Here's how the part is built. I have some questions about the finished solid (model axes, mm). A direction names the side the tool comes from. Round coordinates to 2 decimals unless told otherwise and drop trailing zeros. Order: outer loops, then holes, each group sorted by start corner. A loop starts at its lowest first (then second) coordinate and runs counter-clockwise, first axis right, second up. Notation, with made-up numbers: M -1,-27 L 43,-27 A16 cw 43,4 Z; hole C 84.25,30 d2. An arc over 180 degrees is marked long. Write item = value, one per line. Start each with the question number.
Item 1: I want a section at B-B, the plane y = 3.25. List the corners of the cut face in (x, z) for me.
Item 2: Please list where these lines run through material, in increasing order: L1, parallel to X at y = 0.25, z = -0.25; L2, parallel to X at y = 2.25, z = -4.4; L3, parallel to Z at x = 7.5, y = 3.75.
Item 3: I want a section at A-A, the plane y = -0.5. List the corners of the cut face in (x, z) for me.
Item 4: I want a section at C-C, the plane x = 6.5. List the corners of the cut face in (y, z) for me, plus the area to 3 significant figures.
Item 5: I'm going to push flat-ended pins straight in: P1, Ø0.7, axis at x = 5, y = -0.5, coming from the -Z side; P2, Ø0.7, axis at y = -2, z = -2.5, coming from the +X side. Where does each tip first touch, or does it pass through?
Item 6: We'd pull the mould along Z, two halves only. Please class faces 3 (the face through (9.1, 5, -3)), 4 (the face through (5, 3, 0)), 5 (the face through (1, 0, -3)): pulls with the +Z half, pulls with the -Z half, needs draft (parallel to the pull), parting line crosses it, or undercut.
Item 7: I want a section at D-D, the plane z = -3.8. List the corners of the cut face in (x, y) for me.
Item 8: For faces 1 (the face through (5, 4, -0.8)), 2 (the face through (5, 3, -5.75)), which set-ups out of +Z, -Z, +X, -X, +Y, -Y let a thin tool reach every point of the face, with its end or its side?
```python
from build123d import *

# Parameters (mm, degrees)
SKETCH_1_W                         = 9.9
SKETCH_1_H                         = 5.75
EXTRUDE_1_DEPTH                    = 7
SKETCH_2_W                         = 8.3
SKETCH_2_H                         = 4.15
CUT_EXTRUDE_1_DEPTH                = 5
CUT_EXTRUDE_2_REACH                = 15.419
SKETCH_3_W                         = 1
SKETCH_3_H                         = 0.8
EXTRUDE_START                      = -5.5
SKETCH_4_W                         = 0.64
SKETCH_4_H                         = 0.64
EXTRUDE_2_DEPTH                    = 10.5
CHAMFER_1_SIZE                     = 0.2
PATTERN_LINEAR_4_COUNT             = 3
PATTERN_LINEAR_4_PITCH             = 2.5
CHAMFER_1_OF_PATTERN_LINEAR_4_SIZE = 0.2
CUT_EXTRUDE_3_REACH                = 15.419
CUT_EXTRUDE_4_DEPTH                = 14.419109508
FILLET_1_R                         = 0.1


with BuildPart() as part:
    # Эскиз1 → Бобышка-Вытянуть1 (new body)
    with BuildSketch(Plane(origin=(0, 0, 0), x_dir=(1, 0, 0), z_dir=(0, 1, 0))):
        with Locations((4.95, 2.875)):
            Rectangle(SKETCH_1_W, SKETCH_1_H)
    extrude(amount=EXTRUDE_1_DEPTH)

    # Эскиз2 → Вырез-Вытянуть1 (cut)
    with BuildSketch(Plane(origin=(0, 7, 0), x_dir=(1, 0, 0), z_dir=(0, 1, 0))):
        with Locations((4.95, 2.875)):
            Rectangle(SKETCH_2_W, SKETCH_2_H)
    extrude(amount=-CUT_EXTRUDE_1_DEPTH, mode=Mode.SUBTRACT)

    # Эскиз3 → Вырез-Вытянуть2 (cut, up to next)
    with BuildSketch(Plane.XY, mode=Mode.PRIVATE) as cut_extrude_2_sk1:
        with Locations((2.45, 0.4)):
            Rectangle(SKETCH_3_W, SKETCH_3_H)
    cut_extrude_2_tool1 = extrude(cut_extrude_2_sk1.sketch, amount=-CUT_EXTRUDE_2_REACH, mode=Mode.PRIVATE) & part.part
    # Эскиз3 → Вырез-Вытянуть2 (cut, up to next)
    with BuildSketch(Plane.XY, mode=Mode.PRIVATE) as cut_extrude_2_sk2:
        with Locations((4.95, 0.4)):
            Rectangle(SKETCH_3_W, SKETCH_3_H)
    cut_extrude_2_tool2 = extrude(cut_extrude_2_sk2.sketch, amount=-CUT_EXTRUDE_2_REACH, mode=Mode.PRIVATE) & part.part
    # Эскиз3 → Вырез-Вытянуть2 (cut, up to next)
    with BuildSketch(Plane.XY, mode=Mode.PRIVATE) as cut_extrude_2_sk3:
        with Locations((7.45, 0.4)):
            Rectangle(SKETCH_3_W, SKETCH_3_H)
    cut_extrude_2_tool3 = extrude(cut_extrude_2_sk3.sketch, amount=-CUT_EXTRUDE_2_REACH, mode=Mode.PRIVATE) & part.part
    add(cut_extrude_2_tool1.solids().sort_by_distance((2.45, 0.4, 0))[0], mode=Mode.SUBTRACT)
    add(cut_extrude_2_tool2.solids().sort_by_distance((4.95, 0.4, 0))[0], mode=Mode.SUBTRACT)
    add(cut_extrude_2_tool3.solids().sort_by_distance((7.45, 0.4, 0))[0], mode=Mode.SUBTRACT)

    # Эскиз4 → Бобышка-Вытянуть2 (add)
    with BuildSketch(Plane(origin=(0, 2, 0), x_dir=(1, 0, 0), z_dir=(0, 1, 0)).offset(EXTRUDE_START)):
        with Locations((2.45, 2.64)):
            Rectangle(SKETCH_4_W, SKETCH_4_H)
    extrude_2 = extrude(amount=EXTRUDE_2_DEPTH)

    # Фаска1
    chamfer_1_edges = [part.edges().sort_by_distance(p)[0] for p in [
        (2.13, 7, -2.64),
        (2.13, -3.5, -2.64),
        (2.45, 7, -2.96),
        (2.45, -3.5, -2.96),
        (2.77, 7, -2.64),
        (2.77, -3.5, -2.64),
        (2.45, 7, -2.32),
        (2.45, -3.5, -2.32),
    ]]
    chamfer(chamfer_1_edges, length=CHAMFER_1_SIZE)

    # Линейный массив4: Бобышка-Вытянуть2 ×3
    with Locations(*[(i * PATTERN_LINEAR_4_PITCH, 0, 0) for i in range(1, PATTERN_LINEAR_4_COUNT)]):
        add(extrude_2)

    # Фаска1 of Линейный массив4
    chamfer_1_of_pattern_linear_4_edges = [part.edges().sort_by_distance(p)[0] for p in [
        (4.63, 7, -2.64),
        (4.63, -3.5, -2.64),
        (4.95, 7, -2.96),
        (4.95, -3.5, -2.96),
        (5.27, 7, -2.64),
        (5.27, -3.5, -2.64),
        (4.95, 7, -2.32),
        (4.95, -3.5, -2.32),
        (7.13, 7, -2.64),
        (7.13, -3.5, -2.64),
        (7.45, 7, -2.96),
        (7.45, -3.5, -2.96),
        (7.77, 7, -2.64),
        (7.77, -3.5, -2.64),
        (7.45, 7, -2.32),
        (7.45, -3.5, -2.32),
    ]]
    chamfer(chamfer_1_of_pattern_linear_4_edges, length=CHAMFER_1_OF_PATTERN_LINEAR_4_SIZE)

    # Эскиз5 → Вырез-Вытянуть3 (cut, up to next)
    with BuildSketch(Plane.XY, mode=Mode.PRIVATE) as cut_extrude_3_sk1:
        with BuildLine():
            Line((1.95, 7), (2.95, 7))
            Line((2.95, 7), (2.95, 4))
            Line((2.95, 4), (2.45, 4))
            ThreePointArc((2.45, 4), (2.096446609, 4.146446609), (1.95, 4.5))
            Line((1.95, 4.5), (1.95, 6.153589838))
            ThreePointArc((1.95, 6.153589838), (1.976794919, 6.253589838), (2.05, 6.326794919))
            ThreePointArc((2.05, 6.326794919), (2.15, 6.5), (2.05, 6.673205081))
            ThreePointArc((2.05, 6.673205081), (1.976794919, 6.746410162), (1.95, 6.846410162))
            Line((1.95, 6.846410162), (1.95, 7))
        make_face()
    cut_extrude_3_tool1 = extrude(cut_extrude_3_sk1.sketch, amount=-CUT_EXTRUDE_3_REACH, mode=Mode.PRIVATE) & part.part
    # Эскиз5 → Вырез-Вытянуть3 (cut, up to next)
    with BuildSketch(Plane.XY, mode=Mode.PRIVATE) as cut_extrude_3_sk2:
        with BuildLine():
            Line((6.95, 7), (7.95, 7))
            Line((7.95, 7), (7.95, 6.846410162))
            ThreePointArc((7.95, 6.846410162), (7.923205081, 6.746410162), (7.85, 6.673205081))
            ThreePointArc((7.85, 6.673205081), (7.75, 6.5), (7.85, 6.326794919))
            ThreePointArc((7.85, 6.326794919), (7.923205081, 6.253589838), (7.95, 6.153589838))
            Line((7.95, 6.153589838), (7.95, 4.5))
            ThreePointArc((7.95, 4.5), (7.803553391, 4.146446609), (7.45, 4))
            Line((7.45, 4), (6.95, 4))
            Line((6.95, 4), (6.95, 7))
        make_face()
    cut_extrude_3_tool2 = extrude(cut_extrude_3_sk2.sketch, amount=-CUT_EXTRUDE_3_REACH, mode=Mode.PRIVATE) & part.part
    add(cut_extrude_3_tool1.solids().sort_by_distance((2.467377, 5.501808, 0))[0], mode=Mode.SUBTRACT)
    add(cut_extrude_3_tool2.solids().sort_by_distance((7.432623, 5.501808, 0))[0], mode=Mode.SUBTRACT)

    # Эскиз6 → Вырез-Вытянуть4 (cut, through all)
    with BuildSketch(Plane(origin=(9.9, 0, 0), x_dir=(0, 0, -1), z_dir=(1, 0, 0))):
        with BuildLine():
            Line((0.8, 7), (1.8, 7))
            Line((1.8, 7), (1.8, 4))
            Line((1.8, 4), (1.2, 4))
            ThreePointArc((1.2, 4), (0.917157288, 4.117157288), (0.8, 4.4))
            Line((0.8, 4.4), (0.8, 7))
        make_face()
    extrude(amount=-CUT_EXTRUDE_4_DEPTH, mode=Mode.SUBTRACT)

    # Скругление1
    fillet_1_edges = [part.edges().sort_by_distance(p)[0] for p in [
        (0, 3.5, -5.75),
        (9.9, 3.5, -5.75),
        (9.9, 3.5, 0),
        (0, 3.5, 0),
    ]]
    fillet(fillet_1_edges, radius=FILLET_1_R)


solid = part.part
```
Filled in:
q1.outline = M 0,-5.65 A0.1 ccw 0.1,-5.75 L 9.8,-5.75 A0.1 ccw 9.9,-5.65 L 9.9,-0.1 A0.1 ccw 9.8,0 L 0.1,0 A0.1 ccw 0,-0.1 Z; M 2.13,-2.96 L 2.77,-2.96 L 2.77,-2.32 L 2.13,-2.32 Z; M 4.63,-2.96 L 5.27,-2.96 L 5.27,-2.32 L 4.63,-2.32 Z; M 7.13,-2.96 L 7.77,-2.96 L 7.77,-2.32 L 7.13,-2.32 Z; hole M 0.8,-4.95 L 9.1,-4.95 L 9.1,-0.8 L 0.8,-0.8 Z
q2.L1 = 0 to 1.95, 2.95 to 4.45, 5.45 to 6.95, 7.95 to 9.9
q2.L2 = 0 to 0.8, 9.1 to 9.9
q2.L3 = -5.75 to -4.95, -2.96 to -2.32, -0.8 to 0
q3.outline = M 2.13,-2.96 L 2.77,-2.96 L 2.77,-2.32 L 2.13,-2.32 Z; M 4.63,-2.96 L 5.27,-2.96 L 5.27,-2.32 L 4.63,-2.32 Z; M 7.13,-2.96 L 7.77,-2.96 L 7.77,-2.32 L 7.13,-2.32 Z
q4.outline = M 0,-5.75 L 7,-5.75 L 7,-4.95 L 2,-4.95 L 2,-0.8 L 7,-0.8 L 7,0 L 0,0 Z
q4.area = 19.5 mm^2
q5.P1 = -2.96
q5.P2 = 7.77
q6.face_3 = undercut
q6.face_4 = pulls with the +Z half
q6.face_5 = needs draft
q7.outline = M 0,0 L 1.95,0 L 1.95,0.8 L 2.95,0.8 L 2.95,0 L 4.45,0 L 4.45,0.8 L 5.45,0.8 L 5.45,0 L 6.95,0 L 6.95,0.8 L 7.95,0.8 L 7.95,0 L 9.9,0 L 9.9,7 L 9.1,7 L 9.1,2 L 0.8,2 L 0.8,7 L 0,7 Z
q8.face_1 = +Y
q8.face_2 = -Z, +X, -X, +Y, -Y
